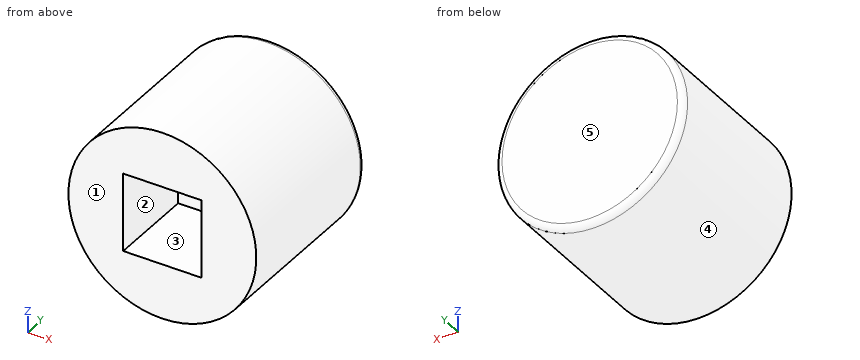
from build123d import *

# Parameters (mm, degrees)
SKETCH1_W          = 3
SKETCH1_H          = 5.5
SKETCH2_W          = 2.5
SKETCH2_H          = 2.5
CUT_EXTRUDE1_DEPTH = 2.8
FILLET1_R          = 0.2


with BuildPart() as part:
    # Sketch1 → Revolve1 (revolve)
    with BuildSketch(Plane(origin=(0, 0, 0), x_dir=(-1, 0, 0), z_dir=(0, 0, -1)), mode=Mode.PRIVATE) as revolve1_sk:
        with Locations((-1.5, 2.75)):
            Rectangle(SKETCH1_W, SKETCH1_H)
    revolve(revolve1_sk.sketch.rotate(Axis((0, 0, 0), (0, 1, 0)), 270), axis=Axis((0, 0, 0), (0, 1, 0)))

    # Sketch2 → Cut-Extrude1 (cut)
    with BuildSketch(Plane.XZ):
        Rectangle(SKETCH2_W, SKETCH2_H)
    extrude(amount=-CUT_EXTRUDE1_DEPTH, mode=Mode.SUBTRACT)

    # Fillet1
    fillet1_edges = [part.edges().sort_by_distance(p)[0] for p in [
        (0, 5.5, -3),
    ]]
    fillet(fillet1_edges, radius=FILLET1_R)


solid = part.part
The model under review builds one solid part; all positions refer to its coordinate system, in mm. Face numbers are marked on the shaded views. A direction names the side the tool comes from. Give positions to 0.01 mm unless a question says otherwise; leave off trailing zeros. Loops run counter-clockwise (first coordinate to the right, second up) from the corner with the lowest first, then second, coordinate; pieces in that order, holes last. Notation, with made-up numbers: (3, -32.5) -> (15, -32.5) arc R31 cw to (15, 4.5) -> close; hole circle Ø2 at (-15.5, 61.5). An arc over 180 degrees is marked (long way). Put each result on its own line as item: value. Start each with the question number.
1. Wall thickness on probe 1 along Y at (x, z) = (-0.5, 1); probe 2 along Z at (x, y) = (0.25, 1.7); probe 3 along X at (y, z) = (2.75, -0.75): over which ranges is each line inside the solid? List them lowest first.
2. For the marked faces 1 and 2, list the 3-axis set-ups (+Z, -Z, +X, -X, +Y, -Y) from which the entire face can be reached by the end or side of a thin tool; tool diameter is ignored.
3. We need section A-A on y = 1.55. State the section outline as (x, z) points.
4. We need section C-C on x = 0. State the section outline as (y, z) points.
5. We need section D-D on y = 4.85. State the section outline as (x, z) points, then the cut area to 3 significant figures.
6. We need section B-B on z = 0. State the section outline as (x, y) points, then the cut area to 3 significant figures.
7. Clearance check with flat-ended pins moving along their axes: P1, Ø0.8, axis at x = 0.5, z = 0.5, coming from the -Y side; P2, Ø1, axis at y = 2.5, z = 1, coming from the -X side; P3, Ø2, axis at x = 2, y = 1.5, coming from the +Z side. State where each tip first meets the part, or that it passes through.
8. Mouldability with a two-part tool opening along Z and no side actions: class the marked faces 3, 4 and 5 as released by +Z, released by -Z, zero draft, split by the parting line, or undercut.
Determined:
1. probe 1: 2.8 to 5.5
1. probe 2: -2.99 to -1.25, 1.25 to 2.99
1. probe 3: -2.9 to -1.25, 1.25 to 2.9
2. face 1: +Z, -Z, +X, -X, -Y
2. face 2: -Y
3. outline: circle Ø6 at (0, 0); hole (-1.25, -1.25) -> (1.25, -1.25) -> (1.25, 1.25) -> (-1.25, 1.25) -> close
4. outline: (0, -3) -> (5.3, -3) arc R0.2 ccw to (5.5, -2.8) -> (5.5, 2.8) arc R0.2 ccw to (5.3, 3) -> (0, 3) -> (0, 1.25) -> (2.8, 1.25) -> (2.8, -1.25) -> (0, -1.25) -> close
5. outline: circle Ø6 at (0, 0)
5. area: 28.3 mm^2
6. outline: (-3, 0) -> (-1.25, 0) -> (-1.25, 2.8) -> (1.25, 2.8) -> (1.25, 0) -> (3, 0) -> (3, 5.3) arc R0.2 ccw to (2.8, 5.5) -> (-2.8, 5.5) arc R0.2 ccw to (-3, 5.3) -> close
6. area: 26.0 mm^2
7. P1: y = 2.8
7. P2: x = -2.96
7. P3: z = 2.83
8. face 3: undercut
8. face 4: split by the parting line
8. face 5: zero draft
